The model under review builds one solid part; all positions refer to its coordinate system, in mm. A direction names the side the tool comes from. Coordinates: 2 decimals unless noted, no trailing zeros. Order: outer loops, then holes, each group sorted by start corner. A loop starts at its lowest first (then second) coordinate and runs counter-clockwise, first axis right, second up. Notation, with made-up numbers: M 3,-24 L 24,-24 A21 ccw 24,-20 Z; hole C 4.5,-28.75 d10. An arc over 180 degrees is marked long. Answer in a Markdown table with one row per item.
from build123d import *

# Parameters (mm, degrees)
BOSS_EXTRUDE1_DEPTH = 6.35


with BuildPart() as part:
    # Sketch1 → Boss-Extrude1 (new body)
    with BuildSketch(Plane.XY):
        with BuildLine():
            Line((3.175, 584.2), (20.193, 584.2))
            Line((20.193, 584.2), (20.193, 574.04))
            Line((20.193, 574.04), (18.288, 574.04))
            Line((18.288, 574.04), (18.288, 572.554033861))
            Line((18.288, 572.554033861), (18.288, 569.976))
            Line((18.288, 569.976), (26.162, 569.976))
            Line((26.162, 569.976), (26.162, 572.554033861))
            Line((26.162, 572.554033861), (26.162, 574.04))
            Line((26.162, 574.04), (24.257, 574.04))
            Line((24.257, 574.04), (24.257, 584.2))
            Line((24.257, 584.2), (41.275, 584.2))
            ThreePointArc((41.275, 584.2), (31.215840751, 558.406178065), (6.35, 546.232522141))
            Line((6.35, 546.232522141), (6.35, 558.8))
            Line((6.35, 558.8), (0, 558.8))
            Line((0, 558.8), (0, 546.232522141))
            ThreePointArc((0, 546.232522141), (-24.865840751, 558.406178065), (-34.925, 584.2))
            Line((-34.925, 584.2), (-17.907, 584.2))
            Line((-17.907, 584.2), (-17.907, 574.04))
            Line((-17.907, 574.04), (-19.812, 574.04))
            Line((-19.812, 574.04), (-19.812, 572.554033861))
            Line((-19.812, 572.554033861), (-19.812, 569.976))
            Line((-19.812, 569.976), (-11.938, 569.976))
            Line((-11.938, 569.976), (-11.938, 572.554033861))
            Line((-11.938, 572.554033861), (-11.938, 574.04))
            Line((-11.938, 574.04), (-13.843, 574.04))
            Line((-13.843, 574.04), (-13.843, 584.2))
            Line((-13.843, 584.2), (3.175, 584.2))
        make_face()
    extrude(amount=BOSS_EXTRUDE1_DEPTH)


solid = part.part
(1) Take a section at A-A (y = 578.5). Write out the cut boundary in (x, z), then the cut area to 3 significant figures.
Report:
| item | result |
|---|---|
| outline | M -34.5,0 L -17.91,0 L -17.91,6.35 L -34.5,6.35 Z; M -13.84,0 L 20.19,0 L 20.19,6.35 L -13.84,6.35 Z; M 24.26,0 L 40.85,0 L 40.85,6.35 L 24.26,6.35 Z |
| area | 427 mm^2 |
(2) Take a section at B-B (z = 1.75). Write out the cut boundary in (x, y) (3 decimals), then the cut area to 3 significant figures.
Report:
| item | result |
|---|---|
| outline | M -34.925,584.2 A38.1 ccw 0,546.233 L 0,558.8 L 6.35,558.8 L 6.35,546.233 A38.1 ccw 41.275,584.2 L 24.257,584.2 L 24.257,574.04 L 26.162,574.04 L 26.162,569.976 L 18.288,569.976 L 18.288,574.04 L 20.193,574.04 L 20.193,584.2 L -13.843,584.2 L -13.843,574.04 L -11.938,574.04 L -11.938,569.976 L -19.812,569.976 L -19.812,574.04 L -17.907,574.04 L -17.907,584.2 Z |
| area | 2,050 mm^2 |
(3) To check wall thickness, follow line 1 (X direction, y = 580, z = 5.5); line 2 (Y direction, x = 18.5, z = 4); line 3 (X direction, y = 581, z = 5.75). State the ranges of each line that lie inside material, in increasing order. Write a range as [from, to].
Report:
| item | result |
|---|---|
| line 1 | [-34.69, -17.91], [-13.84, 20.19], [24.26, 41.04] |
| line 2 | [549.32, 569.98], [574.04, 584.2] |
| line 3 | [-34.79, -17.91], [-13.84, 20.19], [24.26, 41.14] |
(4) The part is to be moulded in two halves that separate along X. For faces 4 (the flat face through (4, 570, 6.35)), 5 (the flat face through (0, 553, 3)), say which applies: +X half, -X half, draft (parallel to the pull), parting line (faces both ways), or undercut.
Report:
| item | result |
|---|---|
| face 4 | draft |
| face 5 | undercut |
(5) Take a section at D-D (x = -9). Write out the cut boundary in (y, z).
Report:
| item | result |
|---|---|
| outline | M 548.1,0 L 584.2,0 L 584.2,6.35 L 548.1,6.35 Z |
(6) Take a section at C-C (y = 554.5). Write out the cut boundary in (x, z).
Report:
| item | result |
|---|---|
| outline | M -20.69,0 L 0,0 L 0,6.35 L -20.69,6.35 Z; M 6.35,0 L 27.04,0 L 27.04,6.35 L 6.35,6.35 Z |
(7) Machinability: for faces 1 (the flat face through (6.35, 552, 3)), 2 (the flat face through (-19, 574.04, 3)), 3 (the flat face through (-17.907, 579, 3)), which of the approach directions +Z, -Z, +X, -X, +Y, -Y give a long, thin tool a straight path to every point of the face, cutting with its end or side? Answer none if there is none.
Report:
| item | result |
|---|---|
| face 1 | +Z, -Z, -Y |
| face 2 | +Z, -Z |
| face 3 | +Z, -Z, +Y |
(8) Insertion check: P1, Ø2, axis at y = 557, z = 4, coming from the -X side; P2, Ø3.5, axis at y = 572, z = 4, coming from the -X side; P3, Ø1.2, axis at y = 571.5, z = 4, coming from the +X side; P4, Ø5, axis at x = -5, y = 565.5, coming from the -Z side. Each pin has a flat end and moves straight along its axis. Give the tip position at first contact, or say it passes through.
Report:
| item | result |
|---|---|
| P1 | x = -24.49 |
| P2 | x = -33.46 |
| P3 | x = 39.3 |
| P4 | z = 0 |
